For this review, take the finished solid that the model builds, in its own axes (mm). A direction names the side the tool comes from. Round coordinates to 2 decimals unless told otherwise and drop trailing zeros. Write each loop counter-clockwise with the first axis right and the second up, starting at its lowest first coordinate (ties: lowest second). Pieces come first, ordered by that corner, then holes.
from build123d import *

# Parameters (mm, degrees)
SKETCH1_W           = 106.68
SKETCH1_H           = 127
BOSS_EXTRUDE1_DEPTH = 3.175
SKETCH2_W           = 4.572
SKETCH2_H           = 55.88
CUT_EXTRUDE1_DEPTH  = 3.175
SKETCH3_W           = 3.81
SKETCH3_H           = 13.0800094
SKETCH3_W_2         = 76.36002
CUT_EXTRUDE2_DEPTH  = 3.175
SKETCH4_R           = 5.999999938
CUT_EXTRUDE3_DEPTH  = 3.175


with BuildPart() as part:
    # Sketch1 → Boss-Extrude1 (new body)
    with BuildSketch(Plane.XY):
        with Locations((15.161716065, 15.987172316)):
            Rectangle(SKETCH1_W, SKETCH1_H)
    extrude(amount=BOSS_EXTRUDE1_DEPTH)

    # Sketch2 → Cut-Extrude1 (cut)
    with BuildSketch(Plane.XY.offset(3.175)):
        with Locations((-9.476283935, 30.973172316)):
            Rectangle(SKETCH2_W, SKETCH2_H)
        with Locations((41.831716065, 30.973172316)):
            Rectangle(SKETCH2_W, SKETCH2_H)
    extrude(amount=-CUT_EXTRUDE1_DEPTH, mode=Mode.SUBTRACT)

    # Sketch3 → Cut-Extrude2 (cut)
    with BuildSketch(Plane.XY.offset(3.175)):
        with Locations((-36.273283935, 72.947167616)):
            Rectangle(SKETCH3_W, SKETCH3_H)
        with Locations((15.161716065, 72.947167616)):
            Rectangle(SKETCH3_W_2, SKETCH3_H)
        with Locations((-36.273283935, -40.972822984)):
            Rectangle(SKETCH3_W, SKETCH3_H)
        with Locations((66.596716065, 72.947167616)):
            Rectangle(SKETCH3_W, SKETCH3_H)
        with Locations((15.161716065, -40.972822984)):
            Rectangle(SKETCH3_W_2, SKETCH3_H)
        with Locations((66.596716065, -40.972822984)):
            Rectangle(SKETCH3_W, SKETCH3_H)
    extrude(amount=-CUT_EXTRUDE2_DEPTH, mode=Mode.SUBTRACT)

    # Sketch4 → Cut-Extrude3 (cut)
    with BuildSketch(Plane.XY.offset(3.175)):
        with Locations((-21.909583935, -15.382818284)):
            Circle(SKETCH4_R)
    extrude(amount=-CUT_EXTRUDE3_DEPTH, mode=Mode.SUBTRACT)


solid = part.part
(1) For line 1 along X through (y, z) = (45, 3.05); line 2 along Y through (x, z) = (-9.5, 0.7); line 3 along Y through (x, z) = (8, 3), list the stretches that pass through material, from the lowest coordinate up.
Geometry check:
line 1: x = -38.18 to -11.76, -7.19 to 39.55, 44.12 to 68.5
line 2: y = -34.43 to 3.03, 58.91 to 66.41
line 3: y = -34.43 to 66.41
(2) We need section D-D, the plane x = 30. Give the boundary of the cut face in (y, z) (3 decimals).
Geometry check:
outline: (-34.433, 0) - (66.407, 0) - (66.407, 3.175) - (-34.433, 3.175) - close
(3) For faces 1 (the face through (42, 3.033, 2)), 2 (the face through (67, 66.407, 2)), 3 (the face through (-36, 66.407, 2)), list the 3-axis set-ups (+Z, -Z, +X, -X, +Y, -Y) from which the entire face can be reached by the end or side of a thin tool; tool diameter is ignored.
Geometry check:
face 1: +Z, -Z
face 2: +Z, -Z, +X, +Y
face 3: +Z, -Z, -X, +Y
(4) We need section B-B, the plane y = 54.5. Give the boundary of the cut face in (x, z) (3 decimals), and give its area (3 significant figures).
Geometry check:
outline: (-38.178, 0) - (-11.762, 0) - (-11.762, 3.175) - (-38.178, 3.175) - close; (-7.19, 0) - (39.546, 0) - (39.546, 3.175) - (-7.19, 3.175) - close; (44.118, 0) - (68.502, 0) - (68.502, 3.175) - (44.118, 3.175) - close
area: 310 mm2
(5) Mouldability with a two-part tool opening along Y and no side actions: class faces 4 (the face through (42, 58.913, 2)), 5 (the face through (15, -34.433, 2)), 6 (the face through (-38.178, 15, 2)) as pulls with the +Y half, pulls with the -Y half, needs draft (parallel to the pull), parting line crosses it, or undercut.
Geometry check:
face 4: undercut
face 5: pulls with the -Y half
face 6: needs draft
(6) For pin 1 Ø1 at (y, z) = (73, 1.5) entering from -X; pin 2 Ø15.5 at (x, y) = (-21.91, -15.38) entering from -Z; pin 3 Ø1 at (x, z) = (41, 1.5) entering from +Y; pin 4 Ø1 at (x, z) = (13, 2) entering from -Y, all flat-tipped, find the tip position at first contact; note any pin that passes through.
Geometry check:
pin 1: stops at x = -34.37
pin 2: stops at z = 0
pin 3: stops at y = 66.41
pin 4: stops at y = -34.43
(7) We need section A-A, the plane y = 69. Give the boundary of the cut face in (x, z) (3 decimals), and give its area (3 significant figures).
Geometry check:
outline: (-34.368, 0) - (-23.018, 0) - (-23.018, 3.175) - (-34.368, 3.175) - close; (53.342, 0) - (64.692, 0) - (64.692, 3.175) - (53.342, 3.175) - close
area: 72.1 mm2
(8) We need section C-C, the plane z = 2.3. State how many separate pieces and enclosed holes the cut face has, and give its area (3 significant figures).
Geometry check:
separate pieces: 1
enclosed holes: 3
area: 10,700 mm2
